Part print with two shaded views. Sizes in mm from the minimum x, y, z corner. A direction names the side the tool comes from. Give positions to 0.01 mm unless a question says otherwise; leave off trailing zeros. Write each loop counter-clockwise with the first axis right and the second up, starting at its lowest first coordinate (ties: lowest second). Pieces come first, ordered by that corner, then holes. Notation, with made-up numbers: (-30, 60) - (-12, 60) arc R24 cw to (-12, 83) - close; hole circle Ø8 at (62, 53). An arc over 180 degrees is marked (long way). One line per item, written item: value. Start each with the question number.
(1) Cut at C-C, the plane x = 30. List the corners of the cut face in (y, z), and give its area (3 significant figures).
(2) Cut at A-A, the plane z = 11.5. List the corners of the cut face in (x, y).
(3) Mould opens along X. For the marked faces 1, 2, 3 and 4 say: pulls with the +X half, pulls with the -X half, needs draft (parallel to the pull), parting line crosses it, or undercut.
(4) Drop a flat-ended pin along its axis: P1, Ø24, axis at x = 20, y = 24, coming from the -Z side. Give the stop position or say it passes through.
(5) Cut at B-B, the plane y = 13. List the corners of the cut face in (x, z), and give its area (3 significant figures).
(6) 3-axis set-ups, long thin cutter, end or side, ignore diameter. For the marked faces 5 and 6: which of +Z, -Z, +X, -X, +Y, -Y reach the whole face in a straight line?
(7) Probe L1, parallel to Z at x = 25, y = 55; L2, parallel to X at y = 9, z = 39. List the from-to ranges inside material, lowest first.
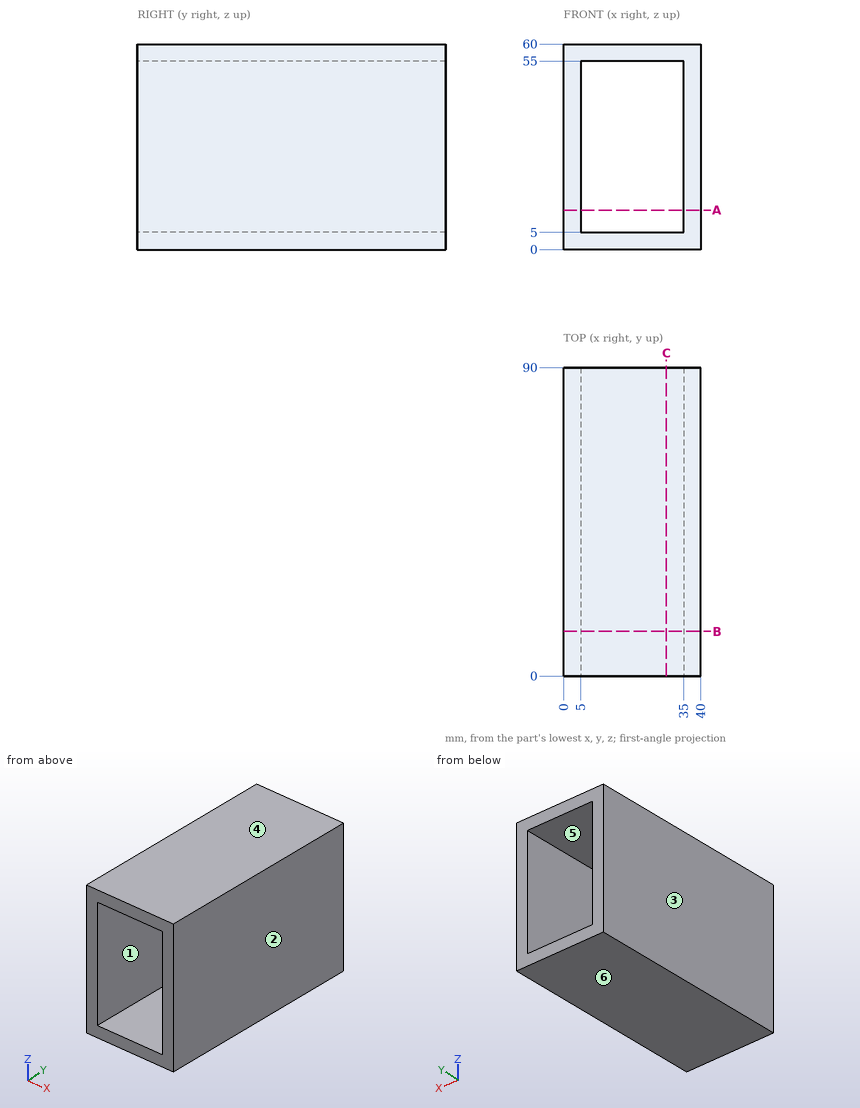
Answers follow:
1. outline: (0, 0) - (90, 0) - (90, 5) - (0, 5) - close; (0, 55) - (90, 55) - (90, 60) - (0, 60) - close
1. area: 900 mm²
2. outline: (0, 0) - (5, 0) - (5, 90) - (0, 90) - close; (35, 0) - (40, 0) - (40, 90) - (35, 90) - close
3. face 1: undercut
3. face 2: pulls with the +X half
3. face 3: pulls with the -X half
3. face 4: needs draft
4. P1: stops at z = 0
5. outline: (0, 0) - (40, 0) - (40, 60) - (0, 60) - close; hole (5, 5) - (35, 5) - (35, 55) - (5, 55) - close
5. area: 900 mm²
6. face 5: +Y, -Y
6. face 6: -Z, +X, -X, +Y, -Y
7. L1: z = 0 to 5, 55 to 60
7. L2: x = 0 to 5, 35 to 40
